from build123d import *

# Parameters (mm, degrees)
SKETCH1_R           = 38.1
SKETCH1_R_2         = 12.7
BOSS_EXTRUDE1_DEPTH = 63.5
SKETCH1_3_R         = 38.1
BOSS_EXTRUDE2_DEPTH = 19.05
SKETCH2_R           = 4.826
BOSS_EXTRUDE3_DEPTH = 19.05
SKETCH2_3_R         = 12.7
CUT_EXTRUDE1_DEPTH  = 12.7


with BuildPart() as part:
    # Sketch1 → Boss-Extrude1 (new body)
    with BuildSketch(Plane.XY):
        Circle(SKETCH1_R)
        Circle(SKETCH1_R_2, mode=Mode.SUBTRACT)
    extrude(amount=BOSS_EXTRUDE1_DEPTH)

    # Sketch1_3 → Boss-Extrude2 (add)
    with BuildSketch(Plane.XY):
        with BuildLine():
            ThreePointArc((44.188017143, -4.81888379), (39.624, 0), (44.188017143, 4.81888379))
            ThreePointArc((44.188017143, 4.81888379), (41.06644522, 17.010278569), (34.653111975, 27.838181163))
            ThreePointArc((34.653111975, 27.838181163), (28.018399098, 28.018399098), (27.838181163, 34.653111975))
            ThreePointArc((27.838181163, 34.653111975), (17.010278569, 41.06644522), (4.81888379, 44.188017143))
            ThreePointArc((4.81888379, 44.188017143), (0, 39.624), (-4.81888379, 44.188017143))
            ThreePointArc((-4.81888379, 44.188017143), (-17.010278569, 41.06644522), (-27.838181163, 34.653111975))
            ThreePointArc((-27.838181163, 34.653111975), (-26.923750994, 33.155980792), (-26.604896424, 31.430896424))
            ThreePointArc((-26.604896424, 31.430896424), (-29.463682181, 27.024044472), (-34.653111975, 27.838181163))
            ThreePointArc((-34.653111975, 27.838181163), (-41.06644522, 17.010278569), (-44.188017143, 4.81888379))
            ThreePointArc((-44.188017143, 4.81888379), (-40.946101795, 3.318580022), (-39.624, 0))
            ThreePointArc((-39.624, 0), (-40.946101795, -3.318580023), (-44.188017143, -4.81888379))
            ThreePointArc((-44.188017143, -4.81888379), (-41.06644522, -17.010278569), (-34.653111975, -27.838181163))
            ThreePointArc((-34.653111975, -27.838181163), (-29.463682181, -27.024044472), (-26.604896424, -31.430896424))
            ThreePointArc((-26.604896424, -31.430896424), (-26.923750994, -33.155980792), (-27.838181163, -34.653111975))
            ThreePointArc((-27.838181163, -34.653111975), (-17.010278569, -41.06644522), (-4.81888379, -44.188017143))
            ThreePointArc((-4.81888379, -44.188017143), (0, -39.624), (4.81888379, -44.188017143))
            ThreePointArc((4.81888379, -44.188017143), (17.010278569, -41.06644522), (27.838181163, -34.653111975))
            ThreePointArc((27.838181163, -34.653111975), (28.018399098, -28.018399098), (34.653111975, -27.838181163))
            ThreePointArc((34.653111975, -27.838181163), (41.06644522, -17.010278569), (44.188017143, -4.81888379))
        make_face()
        Circle(SKETCH1_3_R, mode=Mode.SUBTRACT)
    extrude(amount=BOSS_EXTRUDE2_DEPTH)

    # Sketch2 → Boss-Extrude3 (add)
    with BuildSketch(Plane.XY.offset(63.5)):
        with BuildLine():
            Line((-47.092860393, 19.05), (47.092860393, 19.05))
            ThreePointArc((47.092860393, 19.05), (0, 50.8), (-47.092860393, 19.05))
        make_face()
        with Locations((0, 44.45)):
            Circle(SKETCH2_R, mode=Mode.SUBTRACT)
        with Locations((31.430896424, 31.430896424)):
            Circle(SKETCH2_R, mode=Mode.SUBTRACT)
        with Locations((-31.430896424, 31.430896424)):
            Circle(SKETCH2_R, mode=Mode.SUBTRACT)
        with BuildLine():
            Line((-47.092860393, -19.05), (47.092860393, -19.05))
            ThreePointArc((47.092860393, -19.05), (0, -50.8), (-47.092860393, -19.05))
        make_face()
        with Locations((31.430896424, -31.430896424)):
            Circle(SKETCH2_R, mode=Mode.SUBTRACT)
        with Locations((0, -44.45)):
            Circle(SKETCH2_R, mode=Mode.SUBTRACT)
        with Locations((-31.430896424, -31.430896424)):
            Circle(SKETCH2_R, mode=Mode.SUBTRACT)
    extrude(amount=BOSS_EXTRUDE3_DEPTH)

    # Sketch2_3 → Cut-Extrude1 (cut)
    with BuildSketch(Plane.XY.offset(63.5)):
        with BuildLine():
            Line((32.995567884, 19.05), (-32.995567884, 19.05))
            ThreePointArc((-32.995567884, 19.05), (-38.1, 0), (-32.995567884, -19.05))
            Line((-32.995567884, -19.05), (32.995567884, -19.05))
            ThreePointArc((32.995567884, -19.05), (36.801773982, -9.861005618), (38.1, 0))
            ThreePointArc((38.1, 0), (36.801773982, 9.861005618), (32.995567884, 19.05))
        make_face()
        Circle(SKETCH2_3_R, mode=Mode.SUBTRACT)
    extrude(amount=-CUT_EXTRUDE1_DEPTH, mode=Mode.SUBTRACT)


solid = part.part
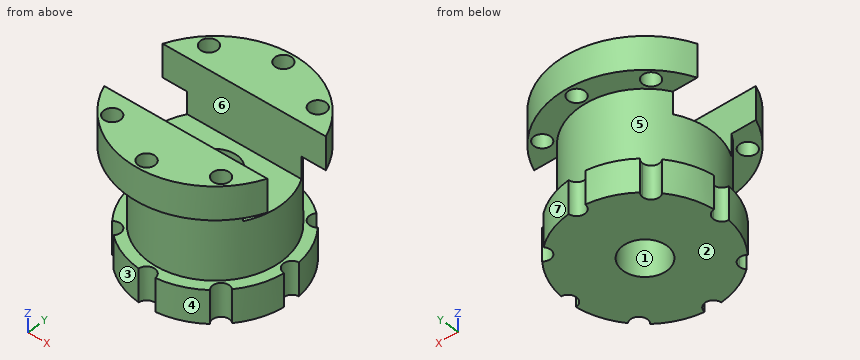
Verification items for the finished model (mm, model axes). Face numbers are marked on the shaded views. A direction names the side the tool comes from. Coordinates: 2 decimals unless noted, no trailing zeros. Order: outer loops, then holes, each group sorted by start corner. A loop starts at its lowest first (then second) coordinate and runs counter-clockwise, first axis right, second up. Notation, with made-up numbers: M 18,-27 L 35,-27 A18 cw 35,-13 Z; hole C 76.5,13.5 d1. An arc over 180 degrees is marked long. One line per item, written item: value. Start each with the question number.
Item 1: Sectioned sample at D-D (y = 22.5). Enter the section's corners in (x, z).
Item 2: Sectioned sample at C-C (y = 10). Enter the section's corners in (x, z).
Item 3: Scan lines: probe 1 along Y at (x, z) = (0.5, 56); probe 2 along Z at (x, y) = (-30.5, -24); probe 3 along Y at (x, z) = (0, 36.5). Record each from-to range of solid material in increasing order.
Item 4: Mould release check, pull along X, two halves, no side actions. Record for the marked faces 1, 2 and 3: released by +X, released by -X, zero draft, split by the parting line, or undercut.
Item 5: Sectioned sample at A-A (z = 71.5). Enter the section's corners in (x, y), then the cut area to 3 significant figures.
Item 6: Gauge pin test, flat ends, axial feed: pin 1 (7.5 mm diameter, centred on x = -31.43, y = -31.43, fed in from -Z); pin 2 (2 mm diameter, centred on x = -18, y = 0, fed in from +Z); pin 3 (12 mm diameter, centred on y = 26, z = 67, fed in from -X); pin 4 (1.5 mm diameter, centred on y = 27.5, z = 10.5, fed in from +X). Record the tip position at first contact, or that the pin passes through.
Item 7: Access from +Z, -Z, +X, -X, +Y, -Y to the whole of each face (thin tool, end or side, straight path). Record for the marked faces 4, 5, 6 and 7.
Item 8: Sectioned sample at B-B (x = 0). Enter the section's corners in (y, z), then the cut area to 3 significant figures.
Conclusion:
1. outline: M -45.55,63.5 L -30.75,63.5 L -30.75,19.05 L -38.33,19.05 L -38.33,0 L 38.33,0 L 38.33,19.05 L 30.75,19.05 L 30.75,63.5 L 45.55,63.5 L 45.55,82.55 L -45.55,82.55 Z
2. outline: M -43.31,0 L -7.83,0 L -7.83,50.8 L -36.76,50.8 L -36.76,19.05 L -43.31,19.05 Z; M 7.83,0 L 43.31,0 L 43.31,19.05 L 36.76,19.05 L 36.76,50.8 L 7.83,50.8 Z
3. probe 1: y = -38.1 to -19.05, 19.05 to 38.1
3. probe 2: z = 0 to 19.05, 63.5 to 82.55
3. probe 3: y = -38.1 to -12.7, 12.7 to 38.1
4. face 1: undercut
4. face 2: zero draft
4. face 3: released by -X
5. outline: M -47.09,-19.05 A50.8 ccw 47.09,-19.05 Z; M -47.09,19.05 L 47.09,19.05 A50.8 ccw Z; hole C -31.43,-31.43 d9.65; hole C -31.43,31.43 d9.65; hole C 0,-44.45 d9.65; hole C 0,44.45 d9.65; hole C 31.43,-31.43 d9.65; hole C 31.43,31.43 d9.65
5. area: 3,890 mm^2
6. pin 1: passes through
6. pin 2: stops at z = 50.8
6. pin 3: stops at x = -46.7
6. pin 4: stops at x = 35.5
7. face 4: -Z, +X, -Y
7. face 5: none
7. face 6: +Z, +X, -X
7. face 7: -Z, +X, +Y
8. outline: M -50.8,63.5 L -49.28,63.5 L -49.28,82.55 L -50.8,82.55 Z; M -39.62,0 L -12.7,0 L -12.7,50.8 L -19.05,50.8 L -19.05,82.55 L -39.62,82.55 L -39.62,63.5 L -38.1,63.5 L -38.1,19.05 L -39.62,19.05 Z; M 12.7,0 L 39.62,0 L 39.62,19.05 L 38.1,19.05 L 38.1,63.5 L 39.62,63.5 L 39.62,82.55 L 19.05,82.55 L 19.05,50.8 L 12.7,50.8 Z; M 49.28,63.5 L 50.8,63.5 L 50.8,82.55 L 49.28,82.55 Z
8. area: 3,960 mm^2
